Verification items for the finished model (mm, model axes). A direction names the side the tool comes from. Give positions to 0.01 mm unless a question says otherwise; leave off trailing zeros. Write each loop counter-clockwise with the first axis right and the second up, starting at its lowest first coordinate (ties: lowest second). Pieces come first, ordered by that corner, then holes. Notation, with made-up numbers: (-21, 16.25) - (21, 16.25) arc R28 cw to (21, 45.25) - close; hole circle Ø2 at (-33.5, 65). An arc over 180 degrees is marked (long way). Put each result on its own line as item: value.
from build123d import *

# Parameters (mm, degrees)
SKETCH1_R           = 7.5
BOSS_EXTRUDE1_DEPTH = 49.5
CHAMFER1_SIZE       = 0.4
SKETCH2_W           = 1.1
SKETCH2_H           = 0.35


with BuildPart() as part:
    # Sketch1 → Boss-Extrude1 (new, symmetric)
    with BuildSketch(Plane(origin=(0, 0, 0), x_dir=(0, 0, -1), z_dir=(1, 0, 0))):
        Circle(SKETCH1_R)
    extrude(amount=BOSS_EXTRUDE1_DEPTH, both=True)

    # Chamfer1
    chamfer1_edges = [part.edges().sort_by_distance(p)[0] for p in [
        (-49.5, 0, 7.5),
        (49.5, 0, 7.5),
    ]]
    chamfer(chamfer1_edges, length=CHAMFER1_SIZE)

    # Sketch2 → Cut-Revolve1 (revolve, cut)
    with BuildSketch(Plane.XY, mode=Mode.PRIVATE) as cut_revolve1_sk:
        with Locations((-3.05, 7.325)):
            Rectangle(SKETCH2_W, SKETCH2_H)
        with Locations((3.05, 7.325)):
            Rectangle(SKETCH2_W, SKETCH2_H)
    revolve(cut_revolve1_sk.sketch.rotate(Axis((0, 0, 0), (-1, 0, 0)), 90), axis=Axis((0, 0, 0), (-1, 0, 0)), mode=Mode.SUBTRACT)


solid = part.part
Q1. Release check for a two-part mould opening along X. For faces 1 (the face through (3.06, -7.09, 0.93)), 2 (the face through (0.035, 0.33, 7.493)), 3 (the face through (49.5, 0, 0)), 4 (the face through (-49.5, 0, 0)) record: released by +X, released by -X, zero draft, split by the parting line, or undercut.
Answers follow:
face 1: undercut
face 2: zero draft
face 3: released by +X
face 4: released by -X
Q2. Set-up check for faces 5 (the face through (-26.032, 0.33, 7.493)), 6 (the face through (-3.04, -7.09, 0.93)): record each of +Z, -Z, +X, -X, +Y, -Y from which the full face is reachable in a straight line by a thin tool's end or side.
Answers follow:
face 5: +X, -X
face 6: none
Q3. Go/stop test with flat-tipped pins: pin 1 Ø1 at (x, y) = (-4, -4) entering from -Z; pin 2 Ø3 at (x, z) = (34.5, 3) entering from -Y; pin 3 Ø4 at (x, z) = (32, -5) entering from +Y. Record where each tip stops, or that it passes through.
Answers follow:
pin 1: stops at z = -6.63
pin 2: stops at y = -7.35
pin 3: stops at y = 6.87
Q4. Section check A-A, the plane x = -23. Record the cut outline in (y, z), plus the area to 3 significant figures.
Answers follow:
outline: circle Ø15 at (0, 0)
area: 177 mm2
Q5. Scan lines: line 1 along Y through (x, z) = (-35.5, 2.25); line 2 along Y through (x, z) = (-26.5, 0.5); line 3 along X through (y, z) = (-2.5, 6.75). Record each from-to range of solid material in increasing order.
Answers follow:
line 1: y = -7.15 to 7.15
line 2: y = -7.48 to 7.48
line 3: x = -49.4 to -3.6, -2.5 to 2.5, 3.6 to 49.4
